The listing builds one solid part. Answer for the finished solid, in the listing's coordinates (mm). Face numbers are marked on the shaded views. A direction names the side the tool comes from. Round coordinates to 2 decimals unless told otherwise and drop trailing zeros. Write each loop counter-clockwise with the first axis right and the second up, starting at its lowest first coordinate (ties: lowest second). Pieces come first, ordered by that corner, then holes.
(1) Find the intervals of material crossed by probe 1 along X at (y, z) = (-9.5, 6.75); probe 2 along X at (y, z) = (-9, 5.5); probe 3 along Y at (x, z) = (3, 14.5), in increasing order.
(2) A cutting plane is placed at C-C, the plane y = -15. Give the vertices of the cut face in (x, z).
(3) A cutting plane is placed at B-B, the plane x = -11. Give the vertices of the cut face in (y, z).
(4) For the marked faces 5 and 6, determine the directions among +Z, -Z, +X, -X, +Y, -Y from which every point of the face is accessible in a straight line to the end or side of a thin tool.
(5) A cutting plane is placed at A-A, the plane y = 0. Give the vertices of the cut face in (x, z).
(6) Each of these flat-tipped pins is pushed along its axis until it touches: pin 1 Ø1.5 at (x, z) = (-14.5, 12) entering from +Y; pin 2 Ø2 at (y, z) = (-14.5, 11) entering from -X; pin 3 Ø12 at (x, y) = (-1.5, 4.5) entering from +Z. Where does it stop, or does it pass through?
(7) The mould has two halves that part along X. Classify the marked faces 1, 2, 3 and 4: +X half, -X half, draft (parallel to the pull), parting line (faces both ways), or undercut.
from build123d import *

# Parameters (mm, degrees)
SKETCH1_R           = 30
BOSS_EXTRUDE1_DEPTH = 15
CUT_EXTRUDE1_DEPTH  = 10
SKETCH3_R           = 2
CUT_EXTRUDE2_DEPTH  = 46


with BuildPart() as part:
    # Sketch1 → Boss-Extrude1 (new body)
    with BuildSketch(Plane.XY):
        Circle(SKETCH1_R)
    extrude(amount=BOSS_EXTRUDE1_DEPTH)

    # Sketch2 → Cut-Extrude1 (cut)
    with BuildSketch(Plane.XY.offset(15)):
        Polygon((0, 14), (-12.124355653, 7), (-12.124355653, -7), (0, -14), (12.124355653, -7), (12.124355653, 7), align=None)
    extrude(amount=-CUT_EXTRUDE1_DEPTH, mode=Mode.SUBTRACT)

    # Sketch3 → Cut-Extrude2 (cut, through all)
    with BuildSketch(Plane(origin=(0, 0, 0), x_dir=(-1, 0, 0), z_dir=(0, 0, -1))):
        with Locations((0, 30)):
            Circle(SKETCH3_R)
        with Locations((7.764571353, 28.977774789)):
            Circle(SKETCH3_R)
        with Locations((15, 25.980762114)):
            Circle(SKETCH3_R)
        with Locations((21.213203436, 21.213203436)):
            Circle(SKETCH3_R)
        with Locations((25.980762114, 15)):
            Circle(SKETCH3_R)
        with Locations((28.977774789, 7.764571353)):
            Circle(SKETCH3_R)
        with Locations((30, 0)):
            Circle(SKETCH3_R)
        with Locations((28.977774789, -7.764571353)):
            Circle(SKETCH3_R)
        with Locations((25.980762114, -15)):
            Circle(SKETCH3_R)
        with Locations((21.213203436, -21.213203436)):
            Circle(SKETCH3_R)
        with Locations((15, -25.980762114)):
            Circle(SKETCH3_R)
        with Locations((7.764571353, -28.977774789)):
            Circle(SKETCH3_R)
        with Locations((0, -30)):
            Circle(SKETCH3_R)
        with Locations((-7.764571353, -28.977774789)):
            Circle(SKETCH3_R)
        with Locations((-15, -25.980762114)):
            Circle(SKETCH3_R)
        with Locations((-21.213203436, -21.213203436)):
            Circle(SKETCH3_R)
        with Locations((-25.980762114, -15)):
            Circle(SKETCH3_R)
        with Locations((-28.977774789, -7.764571353)):
            Circle(SKETCH3_R)
        with Locations((-30, 0)):
            Circle(SKETCH3_R)
        with Locations((-28.977774789, 7.764571353)):
            Circle(SKETCH3_R)
        with Locations((-25.980762114, 15)):
            Circle(SKETCH3_R)
        with Locations((-21.213203436, 21.213203436)):
            Circle(SKETCH3_R)
        with Locations((-15, 25.980762114)):
            Circle(SKETCH3_R)
        with Locations((-7.764571353, 28.977774789)):
            Circle(SKETCH3_R)
    extrude(amount=-CUT_EXTRUDE2_DEPTH, mode=Mode.SUBTRACT)


solid = part.part
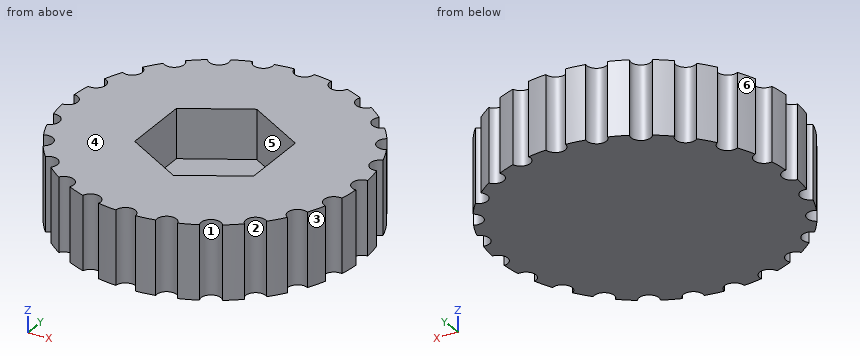
Solutions:
1. probe 1: x = -27.98 to -7.79, 7.79 to 27.98
1. probe 2: x = -27.4 to -8.66, 8.66 to 27.4
1. probe 3: y = -29.85 to -12.27, 12.27 to 29.85
2. outline: (-23.98, 0) - (23.98, 0) - (23.98, 15) - (-23.98, 15) - close
3. outline: (-27.91, 0) - (27.91, 0) - (27.91, 15) - (7.65, 15) - (7.65, 5) - (-7.65, 5) - (-7.65, 15) - (-27.91, 15) - close
4. face 5: +Z
4. face 6: +Z, -Z, -X, +Y
5. outline: (-28, 0) - (28, 0) - (28, 15) - (12.12, 15) - (12.12, 5) - (-12.12, 5) - (-12.12, 15) - (-28, 15) - close
6. pin 1: stops at y = 24.42
6. pin 2: stops at x = -24.66
6. pin 3: stops at z = 5
7. face 1: undercut
7. face 2: undercut
7. face 3: +X half
7. face 4: draft
